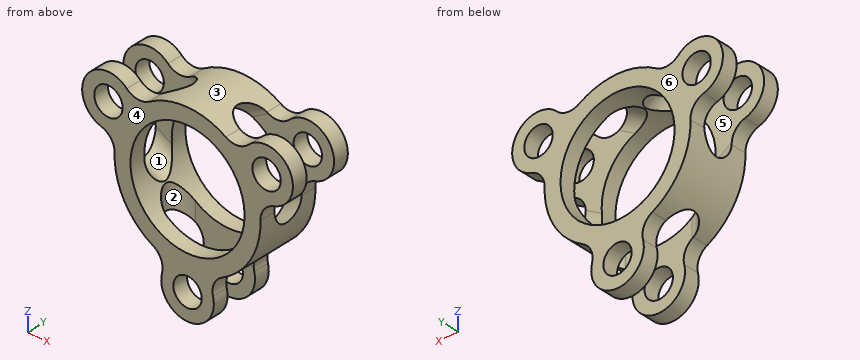
from build123d import *

# Parameters (mm, degrees)
SKETCH_R           = 4.5
SKETCH_R_2         = 18.110743
PAD_DEPTH          = 20
POCKET_DEPTH       = 60
POLARPATTERN_COUNT = 3


with BuildPart() as part:
    # Sketch → Pad (new body)
    with BuildSketch(Plane.XZ):
        with BuildLine():
            ThreePointArc((12.178111, 19.713984), (0, 23.172129), (-12.178111, 19.713984))
            ThreePointArc((-19.292673, 20.489517), (-15.868632, 18.879438), (-12.178111, 19.713984))
            ThreePointArc((-19.292673, 20.489517), (-32.342002, 18.672663), (-27.390779, 6.463187))
            ThreePointArc((-23.161867, 0.689562), (-24.284389, 4.302919), (-27.390779, 6.463187))
            ThreePointArc((-23.161867, 0.689562), (-20.067652, -11.586065), (-10.983754, -20.403546))
            ThreePointArc((-8.098105, -26.952707), (-8.415755, -23.18236), (-10.983754, -20.403546))
            ThreePointArc((-8.098105, -26.952707), (3e-06, -37.345325), (8.098106, -26.952703))
            ThreePointArc((10.983755, -20.403546), (8.415757, -23.182358), (8.098106, -26.952703))
            ThreePointArc((10.983755, -20.403546), (20.067652, -11.586065), (23.161867, 0.689562))
            ThreePointArc((27.390779, 6.463187), (24.284389, 4.302919), (23.161867, 0.689562))
            ThreePointArc((27.390779, 6.463187), (32.342001, 18.672663), (19.292673, 20.489517))
            ThreePointArc((12.178111, 19.713984), (15.868632, 18.879438), (19.292673, 20.489517))
        make_face()
        with Locations((-25.109476, 14.496963)):
            Circle(SKETCH_R, mode=Mode.SUBTRACT)
        with Locations((25.109476, 14.496963)):
            Circle(SKETCH_R, mode=Mode.SUBTRACT)
        with Locations((1e-06, -28.993925)):
            Circle(SKETCH_R, mode=Mode.SUBTRACT)
        Circle(SKETCH_R_2, mode=Mode.SUBTRACT)
    extrude(amount=PAD_DEPTH)

    # Sketch001 → Pocket (cut)
    with BuildSketch(Plane.XY):
        with BuildLine():
            ThreePointArc((-10.534883, -5), (-15.534883, -10), (-10.534883, -15))
            Line((-10.534883, -15), (10.534883, -15))
            ThreePointArc((10.534883, -15), (15.534883, -10), (10.534883, -5))
            Line((10.534883, -5), (-10.534883, -5))
        make_face()
    pocket = extrude(amount=-POCKET_DEPTH, mode=Mode.SUBTRACT)

    # PolarPattern: Pocket ×3 about axis
    polarpattern_axis = Axis((0, 0, 0), (0, 1, 0))
    for i in range(1, POLARPATTERN_COUNT):
        add(pocket.rotate(polarpattern_axis, i * 360 / POLARPATTERN_COUNT), mode=Mode.SUBTRACT)


solid = part.part
Source: CAD feature listing. Evaluate the final solid. Frame: model axes, mm. Face numbers are marked on the shaded views. A direction names the side the tool comes from. Round coordinates to 2 decimals unless told otherwise and drop trailing zeros. Write each loop counter-clockwise with the first axis right and the second up, starting at its lowest first coordinate (ties: lowest second). Pieces come first, ordered by that corner, then holes. Notation, with made-up numbers: M 40.25,22 L 51.25,22 A32 ccw 51.25,59 Z; hole C -11,-9 d4. An arc over 180 degrees is marked long. One line per item, written item: value. Start each with the question number.
Item 1: Section query B-B (x = 25). Return the cut outline in (y, z), plus the area to 3 significant figures.
Item 2: Pin query (flat end, axial travel): pin 1 (5 mm diameter, centred on y = -17.5, z = 2.5, fed in from +X); pin 2 (8 mm diameter, centred on y = -15, z = 3.5, fed in from +X); pin 3 (8 mm diameter, centred on x = 7.5, y = -12, fed in from +Z). Return the tip coordinate at first contact, or that it passes through.
Item 3: Mould query, pull axis Y, two halves, no side actions, for the marked faces 4, 5 and 6. Classes: pulls with the +Y half, pulls with the -Y half, needs draft (parallel to the pull), parting line crosses it, or undercut.
Item 4: Section query A-A (z = -26). Return the cut outline in (x, y), plus the area to 3 significant figures.
Item 5: Section query C-C (y = -2). Return the cut outline in (x, z), plus the area to 3 significant figures.
Item 6: Set-up query: the marked faces 1, 2 and 3. Return all of +Z, -Z, +X, -X, +Y, -Y with unobstructed straight access to the full face (end or side cutting, diameter ignored); none if empty.
Item 7: Section query D-D (z = -19). Return the cut outline in (x, y).
Item 8: Ray query, L1, parallel to Y at x = -25, z = 20; L2, parallel to Z at x = 1, y = -1; L3, parallel to Z at x = 0, y = -14.75. Return the intervals inside material, ascending. Write a range as from..to.
Result set:
1. outline: M -20,5.11 L -15,5.11 L -15,10 L -20,10 Z; M -20,19 L -15,19 L -15,22.85 L -20,22.85 Z; M -5,5.11 L 0,5.11 L 0,10 L -5,10 Z; M -5,19 L 0,19 L 0,22.85 L -5,22.85 Z
1. area: 87.4 mm²
2. pin 1: stops at x = 24.89
2. pin 2: stops at x = 29.67
2. pin 3: stops at z = 22.91
3. face 4: pulls with the -Y half
3. face 5: undercut
3. face 6: pulls with the +Y half
4. outline: M -7.94,-20 L -3.36,-20 L -3.36,-15 L -7.94,-15 Z; M -7.94,-5 L -3.36,-5 L -3.36,0 L -7.94,0 Z; M 3.36,-20 L 7.94,-20 L 7.94,-15 L 3.36,-15 Z; M 3.36,-5 L 7.94,-5 L 7.94,0 L 3.36,0 Z
4. area: 91.6 mm²
5. outline: M -27.39,6.46 A5.82 cw -23.16,0.69 A23.17 ccw -10.98,-20.4 A5.82 cw -8.1,-26.95 A8.35 ccw long 8.1,-26.95 A5.82 cw 10.98,-20.4 A23.17 ccw 23.16,0.69 A5.82 cw 27.39,6.46 A8.35 ccw long 19.29,20.49 A5.82 cw 12.18,19.71 A23.17 ccw -12.18,19.71 A5.82 cw -19.29,20.49 A8.35 ccw long Z; hole C -25.11,14.5 d9; hole C 0,0 d36.22; hole C 0,-28.99 d9; hole C 25.11,14.5 d9
5. area: 1,110 mm²
6. face 1: +Z
6. face 2: -Z
6. face 3: +Z, +Y, -Y
7. outline: M -13.26,-20 L 13.26,-20 L 13.26,-14.19 A5 cw 10.53,-15 L -10.53,-15 A5 cw -13.26,-14.19 Z; M -13.26,-5.81 A5 cw -10.53,-5 L 10.53,-5 A5 cw 13.26,-5.81 L 13.26,0 L -13.26,0 Z
8. L1: y = -20..-15, -5..0
8. L2: z = -37.29..-33.38, -24.61..-18.08, 18.08..23.15
8. L3: z = 18.11..23.17
